Could you check a few things on this drawing? It's one solid part, dimensions in mm from its lowest x, y, z. A direction names the side the tool comes from. Coordinates: 2 decimals unless noted, no trailing zeros. Order: outer loops, then holes, each group sorted by start corner. A loop starts at its lowest first (then second) coordinate and runs counter-clockwise, first axis right, second up. Notation, with made-up numbers: (-27, 16) -> (4, 16) arc R32 cw to (4, 42) -> close; hole circle Ø9 at (58, 29.25). An arc over 180 degrees is marked (long way). Use a Markdown table: item, result. Add a question column.
1. Suppose I cut it at A-A, the plane x = 29.5. List the corners of the cut face in (y, z) for me.
2. For the marked faces 1 and 2, which set-ups out of +Z, -Z, +X, -X, +Y, -Y let a thin tool reach every point of the face, with its end or its side?
3. If I drill on line 1 along X through (y, z) = (5.25, 22.25) (1 decimal); line 2 along Z through (x, y) = (18, 2.5) (1 decimal); line 3 along X through (y, z) = (5.4, 22.25) (1 decimal), over which ranges is the centre line in solid material (lowest first)? Write a range as from..to.
4. Suppose I cut it at B-B, the plane y = 3.25. List the corners of the cut face in (x, z) for me.
5. For pin 1 Ø5 at (x, z) = (42.06, 22.25) entering from +Y; pin 2 Ø5 at (x, z) = (40.5, 45.5) entering from -Y; pin 3 Ø4 at (y, z) = (3, 16) entering from +X, each with a flat end and sliding along its axis, tell me the tip position at first contact or that it passes through.
6. We'd pull the mould along X, two halves only. Please class the marked faces 3, 4 and 5: pulls with the +X half, pulls with the -X half, needs draft (parallel to the pull), parting line crosses it, or undercut.
7. Suppose I cut it at C-C, the plane z = 22.25. State how many separate pieces and enclosed holes the cut face has, then the cut area to 3 significant figures.
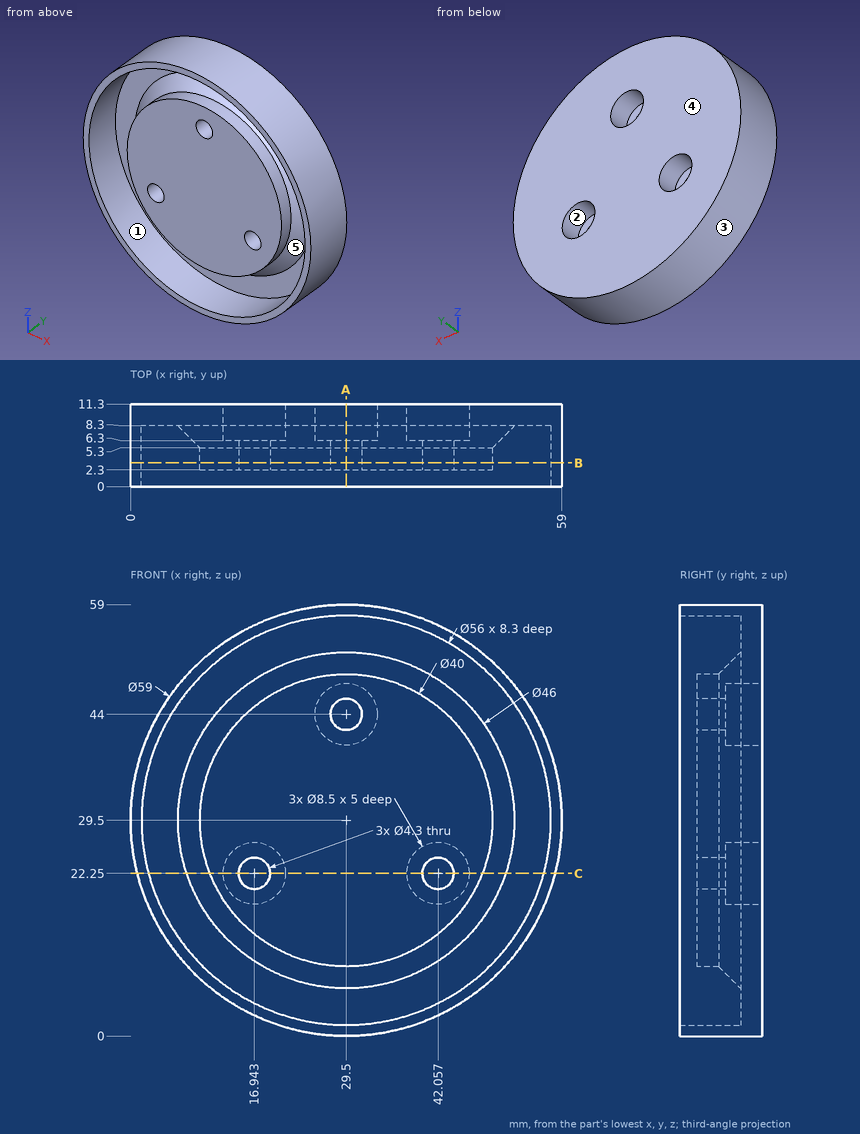
Worked out:
| question | item | result |
|---|---|---|
| 1 | outline | (0, 0) -> (11.3, 0) -> (11.3, 39.75) -> (6.3, 39.75) -> (6.3, 41.85) -> (2.3, 41.85) -> (2.3, 9.5) -> (5.3, 9.5) -> (8.3, 6.5) -> (8.3, 1.5) -> (0, 1.5) -> close; (0, 57.5) -> (8.3, 57.5) -> (8.3, 52.5) -> (5.3, 49.5) -> (2.3, 49.5) -> (2.3, 46.15) -> (6.3, 46.15) -> (6.3, 48.25) -> (11.3, 48.25) -> (11.3, 59) -> (0, 59) -> close |
| 2 | face 1 | -Y |
| 2 | face 2 | +Y |
| 3 | line 1 | x = 0.9..2.5, 10.9..14.8, 19.1..39.9, 44.2..48.1, 56.5..58.1 |
| 3 | line 2 | z = 2.3..4, 13.1..20.4, 24.1..45.9, 55..56.7 |
| 3 | line 3 | x = 0.9..2.5, 10.8..14.8, 19.1..39.9, 44.2..48.2, 56.5..58.1 |
| 4 | outline | circle Ø59 at (29.5, 29.5); circle Ø40 at (29.5, 29.5); hole circle Ø56 at (29.5, 29.5); hole circle Ø4.3 at (16.94, 22.25); hole circle Ø4.3 at (29.5, 44); hole circle Ø4.3 at (42.06, 22.25) |
| 5 | pin 1 | stops at y = 6.3 |
| 5 | pin 2 | stops at y = 2.3 |
| 5 | pin 3 | stops at x = 56.67 |
| 6 | face 3 | parting line crosses it |
| 6 | face 4 | needs draft |
| 6 | face 5 | undercut |
| 7 | separate pieces | 3 |
| 7 | enclosed holes | 0 |
| 7 | area | 311 mm² |
